The model under review builds one solid part; all positions refer to its coordinate system, in mm. Face numbers are marked on the shaded views. A direction names the side the tool comes from. Coordinates: 2 decimals unless noted, no trailing zeros. Loops run counter-clockwise (first coordinate to the right, second up) from the corner with the lowest first, then second, coordinate; pieces in that order, holes last. Notation, with made-up numbers: M 70.5,66 L 95.5,66 A8 ccw 95.5,70 Z; hole C 51,28 d8. An arc over 180 degrees is marked long. One line per item, written item: value.
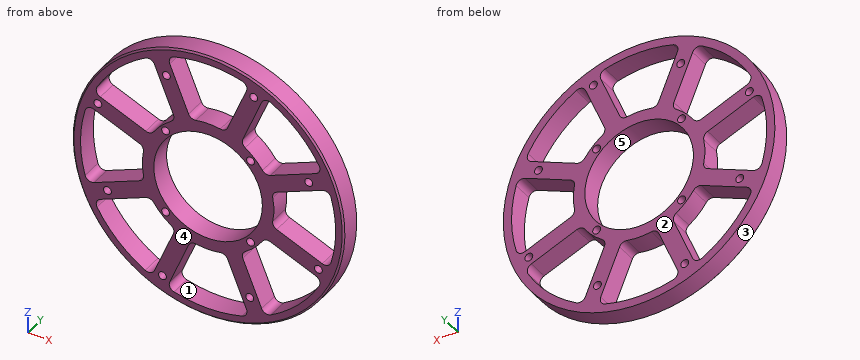
```python
from build123d import *

# Parameters (mm, degrees)
SKETCH2_W                   = 82.55
SKETCH2_H                   = 12.7
F_12_0_189_DIAMETER_HOLE1_D = 4.8006
CIRPATTERN3_COUNT           = 4
CUT_EXTRUDE1_DEPTH          = 13.7
FILLET1_R                   = 4
CIRPATTERN4_COUNT           = 8
FILLET1_OF_CIRPATTERN4_R    = 4
CHAMFER2_SIZE               = 1
SKETCH9_R                   = 33
CUT_EXTRUDE2_DEPTH          = 13.7


with BuildPart() as part:
    # Sketch2 → Revolve1 (revolve)
    with BuildSketch(Plane(origin=(0, 0, 0), x_dir=(0, 0, -1), z_dir=(1, 0, 0))):
        with Locations((-41.275, 6.35)):
            Rectangle(SKETCH2_W, SKETCH2_H)
    revolve(axis=Axis((0, -0.635, 0), (0, 1, 0)))

    # #12 (0.189) Diameter Hole1 (through all)
    with Locations(Plane(origin=(0, 12.7, 0), x_dir=(1, 0, 0), z_dir=(0, 1, 0))):
        with Locations((-27.763683018, 67.027460084), (-61.160825052, 25.333643223), (-25.809397513, 25.809397513)):
            f_12_0_189_diameter_hole1 = Hole(F_12_0_189_DIAMETER_HOLE1_D / 2)

    # CirPattern3: #12 (0.189) Diameter Hole1 ×4 about axis
    cirpattern3_axis = Axis((0, 0, 0), (0, 1, 0))
    for i in range(1, CIRPATTERN3_COUNT):
        add(f_12_0_189_diameter_hole1.rotate(cirpattern3_axis, i * 360 / CIRPATTERN3_COUNT), mode=Mode.SUBTRACT)

    # Sketch8 → Cut-Extrude1 (cut, through all)
    with BuildSketch(Plane(origin=(0, 12.7, 0), x_dir=(1, 0, 0), z_dir=(0, 1, 0))):
        with BuildLine():
            Line((-10.567880231, 38.578749428), (-24.995954941, 73.411203073))
            ThreePointArc((-24.995954941, 73.411203073), (0, 77.55), (24.995954941, 73.411203073))
            Line((24.995954941, 73.411203073), (10.567880231, 38.578749428))
            ThreePointArc((10.567880231, 38.578749428), (0, 40), (-10.567880231, 38.578749428))
        make_face()
    cut_extrude1 = extrude(amount=-CUT_EXTRUDE1_DEPTH, mode=Mode.SUBTRACT)

    # Fillet1
    fillet1_edges = [part.edges().sort_by_distance(p)[0] for p in [
        (10.567880231, 6.35, -38.578749428),
        (-10.567880231, 6.35, -38.578749428),
        (-24.995954941, 6.35, -73.411203073),
        (24.995954941, 6.35, -73.411203073),
    ]]
    fillet(fillet1_edges, radius=FILLET1_R)

    # CirPattern4: Cut-Extrude1 ×8 about axis
    cirpattern4_axis = Axis((0, 0, 0), (0, 1, 0))
    for i in range(1, CIRPATTERN4_COUNT):
        add(cut_extrude1.rotate(cirpattern4_axis, i * 360 / CIRPATTERN4_COUNT), mode=Mode.SUBTRACT)

    # Fillet1 of CirPattern4
    fillet1_of_cirpattern4_edges = [part.edges().sort_by_distance(p)[0] for p in [
        (-19.806675556, 6.35, -34.751915104),
        (-34.751915104, 6.35, -19.806675556),
        (-69.584368749, 6.35, -34.234750266),
        (-34.234750266, 6.35, -69.584368749),
        (-38.578749428, 6.35, -10.567880231),
        (-38.578749428, 6.35, 10.567880231),
        (-73.411203073, 6.35, 24.995954941),
        (-73.411203073, 6.35, -24.995954941),
        (-34.751915104, 6.35, 19.806675556),
        (-19.806675556, 6.35, 34.751915104),
        (-34.234750266, 6.35, 69.584368749),
        (-69.584368749, 6.35, 34.234750266),
        (-10.567880231, 6.35, 38.578749428),
        (10.567880231, 6.35, 38.578749428),
        (24.995954941, 6.35, 73.411203073),
        (-24.995954941, 6.35, 73.411203073),
        (19.806675556, 6.35, 34.751915104),
        (34.751915104, 6.35, 19.806675556),
        (69.584368749, 6.35, 34.234750266),
        (34.234750266, 6.35, 69.584368749),
        (38.578749428, 6.35, 10.567880231),
        (38.578749428, 6.35, -10.567880231),
        (73.411203073, 6.35, -24.995954941),
        (73.411203073, 6.35, 24.995954941),
        (34.751915104, 6.35, -19.806675556),
        (19.806675556, 6.35, -34.751915104),
        (34.234750266, 6.35, -69.584368749),
        (69.584368749, 6.35, -34.234750266),
    ]]
    fillet(fillet1_of_cirpattern4_edges, radius=FILLET1_OF_CIRPATTERN4_R)

    # Chamfer2
    chamfer2_edges = [part.edges().sort_by_distance(p)[0] for p in [
        (0, 0, -82.55),
    ]]
    chamfer(chamfer2_edges, length=CHAMFER2_SIZE)

    # Sketch9 → Cut-Extrude2 (cut, through all)
    with BuildSketch(Plane(origin=(0, 12.7, 0), x_dir=(1, 0, 0), z_dir=(0, 1, 0))):
        Circle(SKETCH9_R)
    extrude(amount=-CUT_EXTRUDE2_DEPTH, mode=Mode.SUBTRACT)


solid = part.part
```
(1) Draft analysis for pull direction Z (two halves, no side actions). For the marked faces 3, 4 and 5, state which applies: pulls with the +Z half, pulls with the -Z half, needs draft (parallel to the pull), parting line crosses it, or undercut.
Checks:
face 3: parting line crosses it
face 4: needs draft
face 5: undercut
(2) Add section B-B on z = 0. State the section outline as (x, y) points, then the cut area to 3 significant figures.
Checks:
outline: M -82.55,1 L -81.55,0 L -77.55,0 L -77.55,12.7 L -82.55,12.7 Z; M -40,0 L -33,0 L -33,12.7 L -40,12.7 Z; M 33,0 L 40,0 L 40,12.7 L 33,12.7 Z; M 77.55,0 L 81.55,0 L 82.55,1 L 82.55,12.7 L 77.55,12.7 Z
area: 304 mm^2
(3) Insertion check: pin 1 Ø1 at (y, z) = (1.5, -62) entering from +X; pin 2 Ø3 at (x, z) = (-27.76, -67.03) entering from -Y; pin 3 Ø6 at (x, z) = (67.03, -27.76) entering from +Y; pin 4 Ø2 at (y, z) = (6.5, -18.5) entering from +X. Each pin has a flat end and moves straight along its axis. Give the tip position at first contact, or say it passes through.
Checks:
pin 1: x = 55.07
pin 2: through
pin 3: y = 12.7
pin 4: x = 80.67
(4) Add section C-C on z = 35.5. State how many separate pieces and enclosed holes the cut face has, then the cut area to 3 significant figures.
Checks:
separate pieces: 3
enclosed holes: 0
area: 697 mm^2
(5) To check wall thickness, follow L1, parallel to Z at x = 19, y = 5.75; L2, parallel to X at y = 11.5, z = -14.5; L3, parallel to Z at x = 52.5, y = 10.25. State the ranges of each line that lie inside material, in increasing order. Write a range as [from, to].
Checks:
L1: [-80.33, -75.19], [-58.94, -26.98], [26.98, 58.94], [75.19, 80.33]
L2: [-81.27, -76.18], [-48.07, -29.64], [29.64, 48.07], [76.18, 81.27]
L3: [-63.7, -57.08], [-27.16, -16.33], [16.33, 27.16], [57.08, 63.7]
(6) Tool access review of the marked faces 1 and 2: name each direction out of +Z, -Z, +X, -X, +Y, -Y from which nothing blocks a thin tool from reaching the whole face with its end or side.
Checks:
face 1: +Y, -Y
face 2: +Z, -Z, +X, -X, +Y
(7) Add section A-A on x = 0. State the section outline as (y, z) points.
Checks:
outline: M 0,-81.55 L 1,-82.55 L 12.7,-82.55 L 12.7,-77.55 L 0,-77.55 Z; M 0,-40 L 12.7,-40 L 12.7,-33 L 0,-33 Z; M 0,33 L 12.7,33 L 12.7,40 L 0,40 Z; M 0,77.55 L 12.7,77.55 L 12.7,82.55 L 1,82.55 L 0,81.55 Z
